```python
from build123d import *

# Parameters (mm, degrees)
SKETCH1_R           = 2.54
SKETCH1_W           = 76.2
SKETCH1_H           = 25.4
BOSS_EXTRUDE1_DEPTH = 3.175
FILLET1_R           = 3.175


with BuildPart() as part:
    # Sketch1 → Boss-Extrude1 (new body)
    # profile 1 of 2: a face of its own
    with BuildSketch(Plane(origin=(0, 0, 0), x_dir=(1, 0, 0), z_dir=(0, 1, 0))):
        Polygon((12.7, 12.7), (-12.7, 12.7), (-12.7, -38.1), (12.7, -38.1), (12.7, -12.7), align=None)
        with Locations(Location((0, -25.4, 0), (0, 0, 270))):
            Circle(SKETCH1_R, mode=Mode.SUBTRACT)
        with Locations(Location((0, 0, 0), (0, 0, 270))):
            Circle(SKETCH1_R, mode=Mode.SUBTRACT)
    # profile 2 of 2: a face of its own
    with BuildSketch(Plane(origin=(0, 0, 0), x_dir=(1, 0, 0), z_dir=(0, 1, 0))):
        with Locations((50.8, 0)):
            Rectangle(SKETCH1_W, SKETCH1_H)
        with Locations(Location((25.4, 0, 0), (0, 0, 270))):
            Circle(SKETCH1_R, mode=Mode.SUBTRACT)
        with Locations(Location((50.8, 0, 0), (0, 0, 270))):
            Circle(SKETCH1_R, mode=Mode.SUBTRACT)
        with Locations(Location((76.2, 0, 0), (0, 0, 270))):
            Circle(SKETCH1_R, mode=Mode.SUBTRACT)
    extrude(amount=BOSS_EXTRUDE1_DEPTH)

    # Fillet1
    fillet1_edges = [part.edges().sort_by_distance(p)[0] for p in [
        (12.7, 1.5875, 38.1),
        (-12.7, 1.5875, 38.1),
        (-12.7, 1.5875, -12.7),
        (88.9, 1.5875, -12.7),
        (88.9, 1.5875, 12.7),
        (12.7, 1.5875, 12.7),
    ]]
    fillet(fillet1_edges, radius=FILLET1_R)


solid = part.part
```
Design review of the part built by this model. Coordinates are the model's own, in mm. A direction names the side the tool comes from. Coordinates: 2 decimals unless noted, no trailing zeros. Order: outer loops, then holes, each group sorted by start corner. A loop starts at its lowest first (then second) coordinate and runs counter-clockwise, first axis right, second up. Notation, with made-up numbers: (31, -25.75) -> (38, -25.75) arc R16 ccw to (38, -16.75) -> close; hole circle Ø4 at (73, 21). An arc over 180 degrees is marked (long way). One line per item, written item: value. Start each with the question number.
Q1. For probe 1 along X at (y, z) = (1.5, 0); probe 2 along X at (y, z) = (0.45, -1); probe 3 along X at (y, z) = (1.75, 25.4), list the stretches that pass through material, from the lowest coordinate up.
Q2. Take a section at D-D, the plane y = 1.85. State the section outline as (x, z) points (3 decimals).
Q3. Take a section at A-A, the plane x = 25.4. State the section outline as (y, z) points (3 decimals), then the cut area to 3 significant figures.
Q4. Insertion check: pin 1 Ø1 at (y, z) = (1, 26) entering from +X; pin 2 Ø4.5 at (x, z) = (0, 0) entering from +Y. Each pin has a flat end and moves straight along its axis. Give the tip position at first contact, or say it passes through.
Q5. Mouldability with a two-part tool opening along Z and no side actions: class faces 1 (the cylindrical face through (13.65, 1.61, 13.61)), 2 (the flat face through (26, 3.175, 7)), 3 (the cylindrical face through (-0.973, 1.565, 27.746)) as pulls with the +Z half, pulls with the -Z half, needs draft (parallel to the pull), parting line crosses it, or undercut.
Q6. Take a section at C-C, the plane x = 0. State the section outline as (y, z) points (3 decimals).
Q7. Take a section at B-B, the plane z = 25.4. State the section outline as (x, y) points (3 decimals).
Q8. Tool access review of faces 4 (the cylindrical face through (2.52, 1.57, -0.33)), 5 (the flat face through (12.7, 2, 26)): name each direction out of +Z, -Z, +X, -X, +Y, -Y from which nothing blocks a thin tool from reaching the whole face with its end or side.
Values follow:
1. probe 1: x = -12.7 to -2.54, 2.54 to 22.86, 27.94 to 48.26, 53.34 to 73.66, 78.74 to 88.9
1. probe 2: x = -12.7 to -2.33, 2.33 to 23.07, 27.73 to 48.47, 53.13 to 73.87, 78.53 to 88.9
1. probe 3: x = -12.7 to -2.54, 2.54 to 12.7
2. outline: (-12.7, -9.525) arc R3.175 ccw to (-9.525, -12.7) -> (85.725, -12.7) arc R3.175 ccw to (88.9, -9.525) -> (88.9, 9.525) arc R3.175 ccw to (85.725, 12.7) -> (15.875, 12.7) arc R3.175 cw to (12.7, 15.875) -> (12.7, 34.925) arc R3.175 ccw to (9.525, 38.1) -> (-9.525, 38.1) arc R3.175 ccw to (-12.7, 34.925) -> close; hole circle Ø5.08 at (0, 0); hole circle Ø5.08 at (0, 25.4); hole circle Ø5.08 at (25.4, 0); hole circle Ø5.08 at (50.8, 0); hole circle Ø5.08 at (76.2, 0)
3. outline: (0, -12.7) -> (3.175, -12.7) -> (3.175, -2.54) -> (0, -2.54) -> close; (0, 2.54) -> (3.175, 2.54) -> (3.175, 12.7) -> (0, 12.7) -> close
3. area: 64.5 mm2
4. pin 1: stops at x = 12.7
4. pin 2: passes through
5. face 1: pulls with the +Z half
5. face 2: needs draft
5. face 3: undercut
6. outline: (0, -12.7) -> (3.175, -12.7) -> (3.175, -2.54) -> (0, -2.54) -> close; (0, 2.54) -> (3.175, 2.54) -> (3.175, 22.86) -> (0, 22.86) -> close; (0, 27.94) -> (3.175, 27.94) -> (3.175, 38.1) -> (0, 38.1) -> close
7. outline: (-12.7, 0) -> (-2.54, 0) -> (-2.54, 3.175) -> (-12.7, 3.175) -> close; (2.54, 0) -> (12.7, 0) -> (12.7, 3.175) -> (2.54, 3.175) -> close
8. face 4: +Y, -Y
8. face 5: +Z, +X, +Y, -Y
